Input: part model. Units: mm. Frame: model coordinates. Give positions to 0.01 mm unless a question says otherwise; leave off trailing zeros. Loops run counter-clockwise (first coordinate to the right, second up) from the corner with the lowest first, then second, coordinate; pieces in that order, holes last. Notation, with made-up numbers: (65, 84.25) - (101, 84.25) arc R23 ccw to (101, 117.25) - close; hole circle Ø7 at (-18.75, 7). An arc over 180 degrees is marked (long way). Answer as a JSON object with one key per item and string values. Group by question number.
(1) Section query C-C (y = 755). Return loops of the section in (x, z), plus the area to 3 significant figures.
(2) Section query D-D (z = 0.65). Return loops of the section in (x, y).
(3) Mould query, pull axis X, two halves, no side actions, for faces 1 (the flat face through (-13, 761, 2)), 2 (the flat face through (-5, 753, 0)), 3 (the conical face through (-2.9, 769.4, 2.1)). Classes: +X half, -X half, draft (parallel to the pull), parting line (faces both ways), or undercut.
(4) Section query A-A (x = -3). Return loops of the section in (y, z), plus the area to 3 significant figures.
(5) Material intervals for L1, parallel to Y at x = -3, z = 1.5; L2, parallel to X at y = 767, z = 0.7; L3, parallel to Y at x = -2.75, z = 3.7, sorted ascending.
(6) Section query B-B (z = 3.6). Return loops of the section in (x, y), plus the area to 3 significant figures.
(7) Pin query (flat end, axial travel): P1, Ø7, axis at x = -3, y = 767, coming from the -Z side; P2, Ø4.5, axis at x = -3, y = 740, coming from the -Z side. Return the tip coordinate at first contact, or that it passes through.
Autodesk Inventor part; units mm, degrees
ref_plane "YZ Plane" through (0, 0, 0) normal (1, 0, 0) x (0, 1, 0)
ref_plane "XZ Plane" through (0, 0, 0) normal (0, 1, 0) x (-1, 0, 0)
ref_plane "XY Plane" through (0, 0, 0) normal (0, 0, 1) x (1, 0, 0)
ref_plane "Work Plane1" through (0, 0, 0) normal (0, 0, 1) x (1, 0, 0)
sketch "Sketch1" plane through (0, 0, 0) normal (0, 0, 1) x (1, 0, 0)
  circle A0 centre (-3, 740) radius 5.2
  circle A1 centre (-3, 767) radius 4.3
  circle A2 centre (-3, 755) radius 4.3
  line L0 (7, 772) -> (7, 750)
  line L1 (7, 750) -> (3.1945, 738.0305)
  arc A3 (-9.1945, 738.0305) -> (3.1945, 738.0305) centre (-3, 740) ccw
  line L2 (-9.1945, 738.0305) -> (-13, 750)
  line L3 (-13, 750) -> (-13, 772)
  line L4 (-13, 772) -> (7, 772)
  point P0 (0, 0)
extrude "Extrusion1" add sketch "Sketch1" along normal blind 4 contours A0 | A1 | A2 | L0 L1 A3 L2 L3 L4
hole "Hole1" at (-3, 740, 0) direction (0, 0, 1) diameter 5.5 end through all
sketch "Sketch2" plane through (0, 0, 4) normal (0, 0, 1) x (1, 0, 0)
  circle A0 centre (-3, 740) radius 5.2
  circle A1 centre (-3, 767) radius 4.3
  circle A2 centre (-3, 755) radius 4.3
  line L0 (7, 772) -> (7, 750)
  line L1 (7, 750) -> (3.1945, 738.0305)
  arc A3 (-9.1945, 738.0305) -> (3.1945, 738.0305) centre (-3, 740) ccw
  line L2 (-9.1945, 738.0305) -> (-13, 750)
  line L3 (-13, 750) -> (-13, 772)
  line L4 (-13, 772) -> (7, 772)
  point P0 (0, 0)
hole "Hole2" at (-3, 767, 4) at (-3, 755, 4) direction (0, 0, -1) diameter 4.5 end through all countersink diameter 8.6 countersink angle 90
properties part number "belt_tentioner_2"
Recorded:
{
 "1": {"outline": "(-13, 0) - (-5.25, 0) - (-5.25, 1.95) - (-7.3, 4) - (-13, 4) - close; (-0.75, 0) - (7, 0) - (7, 4) - (1.3, 4) - (-0.75, 1.95) - close", "area": "57.8 mm^2"},
 "2": {"outline": "(-13, 750) - (-9.19, 738.03) arc R6.5 ccw to (3.19, 738.03) - (7, 750) - (7, 772) - (-13, 772) - close; hole circle Ø5.5 at (-3, 740); hole circle Ø4.5 at (-3, 755); hole circle Ø4.5 at (-3, 767)"},
 "3": {"face 1": "-X half", "face 2": "draft", "face 3": "undercut"},
 "4": {"outline": "(733.5, 0) - (737.25, 0) - (737.25, 4) - (733.5, 4) - close; (742.75, 0) - (752.75, 0) - (752.75, 1.95) - (750.7, 4) - (742.75, 4) - close; (757.25, 0) - (764.75, 0) - (764.75, 1.95) - (762.7, 4) - (759.3, 4) - (757.25, 1.95) - close; (769.25, 0) - (772, 0) - (772, 4) - (771.3, 4) - (769.25, 1.95) - close", "area": "87.6 mm^2"},
 "5": {"L1": "y = 733.5 to 737.25, 742.75 to 752.75, 757.25 to 764.75, 769.25 to 772", "L2": "x = -13 to -5.25, -0.75 to 7", "L3": "y = 733.5 to 737.26, 742.74 to 751.01, 758.99 to 763.01, 770.99 to 772"},
 "6": {"outline": "(-13, 750) - (-9.19, 738.03) arc R6.5 ccw to (3.19, 738.03) - (7, 750) - (7, 772) - (-13, 772) - close; hole circle Ø7.8 at (-3, 755); hole circle Ø7.8 at (-3, 767); hole circle Ø5.5 at (-3, 740)", "area": "556 mm^2"},
 "7": {"P1": "stops at z = 0", "P2": "passes through"}
}
